```python
from build123d import *

# Parameters (mm, degrees)
F1_DEPTH       = 5
F3_D           = 7
F3_CBORE_D     = 12
F3_CBORE_DEPTH = 2


with BuildPart() as f1:
    # F0 (on Top) → F1 (new body)
    with BuildSketch(Plane.XY):
        Polygon((243, 240), (-243, 240), (-243, 198), (-325, 198), (-325, -198), (-243, -198), (-243, -240), (243, -240), (243, -198), (325, -198), (325, 198), (243, 198), align=None)
    extrude(amount=F1_DEPTH)

    # F3 (through all)
    with Locations(Plane.XY.offset(5)):
        with Locations((-163, 220), (-163, -220), (163, -220), (163, 220)):
            CounterBoreHole(F3_D / 2, F3_CBORE_D / 2, F3_CBORE_DEPTH)


solid = f1.part
```
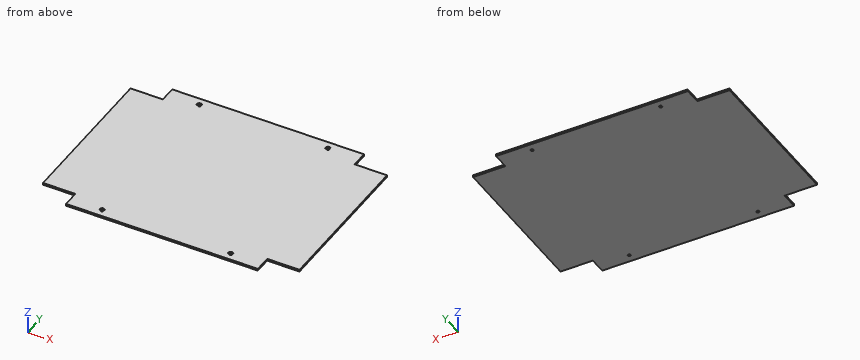
Here's how the part is built. I have some questions about the finished solid (model axes, mm). Give positions to 0.01 mm unless a question says otherwise; leave off trailing zeros. Order: outer loops, then holes, each group sorted by start corner. A loop starts at its lowest first (then second) coordinate and runs counter-clockwise, first axis right, second up. Notation, with made-up numbers: (-35.5, 18.5) -> (-30.5, 18.5) arc R29 cw to (-30.5, 52.5) -> close; hole circle Ø4 at (14.25, -38.5). An arc over 180 degrees is marked (long way). Use CSV: the item, a comma, the result in double quotes. Start each with the question number.
Item 1: If I drill on probe 1 along X at (y, z) = (220.5, 2.8); probe 2 along Y at (x, z) = (163, 0.65); probe 3 along Y at (x, z) = (-163, 4.1), over which ranges is the centre line in solid material (lowest first)? Write a range as [from, to].
Item 2: Suppose I cut it at A-A (y = -206.5). List the corners of the cut face in (x, z) for me.
Item 3: I'm going to push flat-ended pins straight in: P1, Ø6, axis at x = -161.5, y = -219, coming from the +Z side; P2, Ø9.5, axis at x = -163, y = 220, coming from the -Z side; P3, Ø1.5, axis at x = 297, z = 2.5, coming from the +Y side; P4, Ø2.5, axis at y = 208.5, z = 2.5, coming from the +X side. Where does each tip first touch, or does it pass through?
Answer block:
1,probe 1,"x = [-243, -166.46], [-159.54, 159.54], [166.46, 243]"
1,probe 2,"y = [-240, -223.5], [-216.5, 216.5], [223.5, 240]"
1,probe 3,"y = [-240, -226], [-214, 214], [226, 240]"
2,outline,"(-243, 0) -> (243, 0) -> (243, 5) -> (-243, 5) -> close"
3,P1,"stops at z = 3"
3,P2,"stops at z = 0"
3,P3,"stops at y = 198"
3,P4,"stops at x = 243"
